Verification items for the finished model (mm, model axes). Face numbers are marked on the shaded views. Coordinates: 2 decimals unless noted, no trailing zeros. Order: outer loops, then holes, each group sorted by start corner. A loop starts at its lowest first (then second) coordinate and runs counter-clockwise, first axis right, second up.
Q1. Thickness scan on line 1 (X direction, y = 0.75, z = 17); line 2 (Z direction, x = -138, y = 3); line 3 (Z direction, x = -15.5, y = 1.5). Record the ranges inside material, lowest first.
Q2. Depth check by flat-ended pin: P1, Ø1.2, axis at x = -3, y = 3.5, coming from the +Z side; P2, Ø1.9, axis at x = -1.5, y = 4.5, coming from the +Z side; P3, Ø1, axis at x = -153, y = 3.5, coming from the -Z side. Enter the tip coordinate at first touch or a pass-through.
Q3. Draft check along Z on the marked faces 1 and 2. Enter one of: pulls with the +Z half, pulls with the -Z half, needs draft (parallel to the pull), parting line crosses it, or undercut.
Q4. Cross-section at A-A, the plane x = -97. Record the boundary of the cut face in (y, z).
from build123d import *

# Parameters (mm, degrees)
P_IDAT_VYSUNUT_M1_DEPTH  = 8
ODEBRAT_VYSUNUT_M1_DEPTH = 161.106285011
SKICA6_W                 = 16
SKICA6_H                 = 8
P_IDAT_VYSUNUT_M3_DEPTH  = 8
ODEBRAT_VYSUNUT_M4_DEPTH = 161.106285011
SKICA4_W                 = 2.4
SKICA4_H                 = 2.4
ODEBRAT_VYSUNUT_M2_DEPTH = 4.4
SKICA5_W                 = 2
SKICA5_H                 = 2
P_IDAT_VYSUNUT_M2_DEPTH  = 4
ODEBRAT_VYSUNUT_M5_DEPTH = 164.863426365
SKICA12_R                = 2.2
ODEBRAT_VYSUNUT_M7_DEPTH = 9.4


with BuildPart() as part:
    # Skica1 → Přidat vysunutím1 (new body)
    with BuildSketch(Plane(origin=(0, 0, 0), x_dir=(1, 0, 0), z_dir=(0, 1, 0))):
        Polygon((0, 0), (0, -55), (-150.15, -27.472114866), (-150.15, 0), (-142.85, 0), (-142.85, -21.185463454), (-7.3, -46.036644473), (-7.3, 0), align=None)
    extrude(amount=P_IDAT_VYSUNUT_M1_DEPTH)

    # Skica3 → Odebrat vysunutím1 (cut, through all)
    with BuildSketch(Plane(origin=(0, 8, 0), x_dir=(1, 0, 0), z_dir=(0, 1, 0))):
        Polygon((-1, -43.6), (-3.2, -41.6), (-3.2, -48), (-1, -46), (0, -46), (0, -43.6), align=None)
    extrude(amount=-ODEBRAT_VYSUNUT_M1_DEPTH, mode=Mode.SUBTRACT)

    # Skica6 → Přidat vysunutím3 (add)
    with BuildSketch(Plane(origin=(0, 8, 0), x_dir=(1, 0, 0), z_dir=(0, 1, 0))):
        with Locations((-142.15, -4)):
            Rectangle(SKICA6_W, SKICA6_H)
        with Locations((-8, -4)):
            Rectangle(SKICA6_W, SKICA6_H)
    extrude(amount=-P_IDAT_VYSUNUT_M3_DEPTH)

    # Skica9 → Odebrat vysunutím4 (cut, through all)
    with BuildSketch(Plane.XZ):
        Polygon((-142.85, 8), (-134.15, 8), (-134.15, 0), align=None)
        Polygon((-16, 8), (-7.3, 8), (-16, 0), align=None)
    extrude(amount=-ODEBRAT_VYSUNUT_M4_DEPTH, mode=Mode.SUBTRACT)

    # Skica4 → Odebrat vysunutím2 (cut)
    with BuildSketch(Plane(origin=(0, 0, 0), x_dir=(0, 0, -1), z_dir=(1, 0, 0))):
        with Locations((-34.1, 4)):
            Rectangle(SKICA4_W, SKICA4_H)
        with Locations((-13.3, 4)):
            Rectangle(SKICA4_W, SKICA4_H)
    extrude(amount=-ODEBRAT_VYSUNUT_M2_DEPTH, mode=Mode.SUBTRACT)

    # Skica5 → Přidat vysunutím2 (add)
    with BuildSketch(Plane.ZY.offset(150.15)):
        with Locations((13.2, 4)):
            Rectangle(SKICA5_W, SKICA5_H)
    extrude(amount=P_IDAT_VYSUNUT_M2_DEPTH)

    # Skica10 → Odebrat vysunutím5 (cut, through all)
    with BuildSketch(Plane(origin=(0, 8, 0), x_dir=(1, 0, 0), z_dir=(0, 1, 0))):
        Polygon((-150.15, -22.4), (-149.15, -22.4), (-146.95, -24.4), (-146.95, -18), (-149.15, -20), (-150.15, -20), align=None)
    extrude(amount=-ODEBRAT_VYSUNUT_M5_DEPTH, mode=Mode.SUBTRACT)

    # Skica12 → Odebrat vysunutím7 (cut)
    with BuildSketch(Plane(origin=(0, 0, 0), x_dir=(-1, 0, 0), z_dir=(0, 0, -1))):
        with Locations((3.65, 4)):
            Circle(SKICA12_R)
        with Locations((146.5, 4)):
            Circle(SKICA12_R)
    extrude(amount=-ODEBRAT_VYSUNUT_M7_DEPTH, mode=Mode.SUBTRACT)


solid = part.part
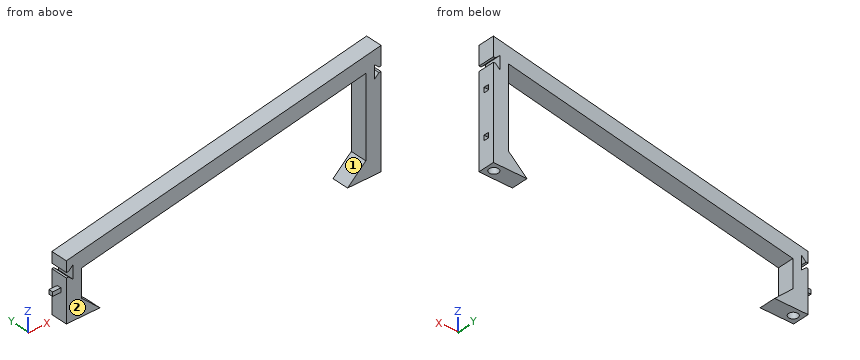
Check values:
1. line 1: x = -150.15 to -142.85, -7.3 to 0
1. line 2: z = 0 to 3.54, 22.07 to 29.7
1. line 3: z = 0 to 0.46, 44.53 to 52.16
2. P1: stops at z = 54.56
2. P2: stops at z = 54.9
2. P3: stops at z = 12.2
3. face 1: undercut
3. face 2: needs draft
4. outline: (0, 29.59) - (8, 29.59) - (8, 37.22) - (0, 37.22) - close
